```python
from build123d import *

# Parameters (mm, degrees)
SKETCH1_R           = 1.9325
BOSS_EXTRUDE1_DEPTH = 112.316
SKETCH2_R           = 3.730040454
BOSS_EXTRUDE2_DEPTH = 0.001
DOME1_FACE_RADIUS   = 3.730040454
DOME1_HEIGHT        = 3
SCALE1_SCALE        = 1.5
SKETCH3_R           = 2.89875
CUT_EXTRUDE1_DEPTH  = 59.7
CHAMFER1_SIZE       = 0.3


with BuildPart() as part:
    # Sketch1 → Boss-Extrude1 (new body)
    with BuildSketch(Plane.XY):
        with Locations(Location((0, 0, 0), (0, 0, 180))):
            Circle(SKETCH1_R)
    extrude(amount=BOSS_EXTRUDE1_DEPTH)

    # Sketch2 → Boss-Extrude2 (add)
    with BuildSketch(Plane.XY.offset(112.316)):
        Circle(SKETCH2_R)
    extrude(amount=BOSS_EXTRUDE2_DEPTH)

    # Dome1: a dome of height H over a round flat face of radius A is a cap of a sphere of radius (A * A + H * H) / (2 * H)
    dome1_r = (DOME1_FACE_RADIUS * DOME1_FACE_RADIUS + DOME1_HEIGHT * DOME1_HEIGHT) / (2 * DOME1_HEIGHT)
    dome1_base = Plane((0, 0, 112.317), z_dir=(0, 0, 1))
    with Locations(dome1_base.offset(DOME1_HEIGHT - dome1_r)):
        dome1_ball = Sphere(dome1_r, mode=Mode.PRIVATE)
    add(split(dome1_ball, bisect_by=dome1_base, keep=Keep.TOP, mode=Mode.PRIVATE))


with BuildPart() as part_1:
    # Scale1: scaled about (0, 0, 59.424709499)
    add(part.part.scale(SCALE1_SCALE).moved(Location((0, 0, -29.71235475))))

    # Sketch3 → Cut-Extrude1 (cut)
    with BuildSketch(Plane(origin=(0, 0, -29.712354749), x_dir=(-1, 0, 0), z_dir=(0, 0, -1))):
        Circle(SKETCH3_R)
    extrude(amount=-CUT_EXTRUDE1_DEPTH, mode=Mode.SUBTRACT)

    # Chamfer1
    chamfer1_edges = [part_1.edges().sort_by_distance(p)[0] for p in [
        (2.89875, 0, 29.987645251),
    ]]
    chamfer(chamfer1_edges, length=CHAMFER1_SIZE)


solid = part_1.part
```
Design review of the part built by this model. Coordinates are the model's own, in mm. A direction names the side the tool comes from. Coordinates: 2 decimals unless noted, no trailing zeros. Order: outer loops, then holes, each group sorted by start corner. A loop starts at its lowest first (then second) coordinate and runs counter-clockwise, first axis right, second up.
1) For faces 1 (the flat face through (0, 0, 29.988)), 2 (the flat face through (2.4, -2.4, 138.762)), list the 3-axis set-ups (+Z, -Z, +X, -X, +Y, -Y) from which the entire face can be reached by the end or side of a thin tool; tool diameter is ignored.
2) Take a section at C-C, the plane z = 89. Give the boundary of the cut face in (x, y).
3) Wall thickness on line 1 along X through (y, z) = (0, 70.5); line 2 along Z through (x, y) = (-1, -3); line 3 along X through (y, z) = (2.25, 133): over which ranges is each line inside the solid? List them lowest first.
4) Clearance check with flat-ended pins moving along their axes: pin 1 (1 mm diameter, centred on x = -2, z = 88, fed in from +Y); pin 2 (2 mm diameter, centred on x = 2, z = 48.5, fed in from +Y); pin 3 (3 mm diameter, centred on x = 2, y = -0.5, fed in from +Z). State where each tip first meets the part, or that it passes through.
Returned:
1. face 1: -Z, +X, -X, +Y, -Y
1. face 2: -Z
2. outline: circle Ø5.8 at (0, 0)
3. line 1: x = -2.9 to 2.9
3. line 2: z = 138.76 to 142.31
3. line 3: x = -1.83 to 1.83
4. pin 1: stops at y = 2.48
4. pin 2: stops at y = 2.72
4. pin 3: stops at z = 143.24
